Design review of the part built by this model. Coordinates are the model's own, in mm. A direction names the side the tool comes from. Round coordinates to 2 decimals unless told otherwise and drop trailing zeros. Order: outer loops, then holes, each group sorted by start corner. A loop starts at its lowest first (then second) coordinate and runs counter-clockwise, first axis right, second up.
from build123d import *

# Parameters (mm, degrees)
SKETCH1_W = 25
SKETCH1_H = 3
SKETCH4_W = 0.74
SKETCH4_H = 0.5
SKETCH5_W = 0.74
SKETCH5_H = 0.5


with BuildPart() as part:
    # Sketch1 → Revolve1 (revolve)
    with BuildSketch(Plane.XY):
        with Locations((0, 1.5)):
            Rectangle(SKETCH1_W, SKETCH1_H)
    revolve(axis=Axis((12.5, 0, 0), (-1, 0, 0)))

    # Sketch2 → Cut-Revolve1 (revolve, cut)
    with BuildSketch(Plane.XY):
        Polygon((11.75, 3), (12.5, 2.25), (12.5, 3), align=None)
    revolve(axis=Axis((12.5, 0, 0), (-1, 0, 0)), mode=Mode.SUBTRACT)

    # Sketch3 → Cut-Revolve2 (revolve, cut)
    with BuildSketch(Plane.XY):
        Polygon((-12.5, 2.25), (-11.75, 3), (-12.5, 3), align=None)
    revolve(axis=Axis((12.5, 0, 0), (-1, 0, 0)), mode=Mode.SUBTRACT)

    # Sketch4 → Cut-Revolve3 (revolve, cut)
    with BuildSketch(Plane.XY):
        with Locations((9.87, 2.75)):
            Rectangle(SKETCH4_W, SKETCH4_H)
    revolve(axis=Axis((12.5, 0, 0), (-1, 0, 0)), mode=Mode.SUBTRACT)

    # Sketch5 → Cut-Revolve4 (revolve, cut)
    with BuildSketch(Plane.XY):
        with Locations((-9.87, 2.75)):
            Rectangle(SKETCH5_W, SKETCH5_H)
    revolve(axis=Axis((12.5, 0, 0), (-1, 0, 0)), mode=Mode.SUBTRACT)


solid = part.part
1) To check wall thickness, follow line 1 along X through (y, z) = (-2.6, 1.3); line 2 along X through (y, z) = (1.75, -2); line 3 along Z through (x, y) = (-9.25, -2.35). State the ranges of each line that lie inside material, in increasing order.
Results:
line 1: x = -11.84 to -10.24, -9.5 to 9.5, 10.24 to 11.84
line 2: x = -12.09 to -10.24, -9.5 to 9.5, 10.24 to 12.09
line 3: z = -1.86 to 1.86
2) Clearance check with flat-ended pins moving along their axes: P1, Ø1, axis at x = -1, y = 1, coming from the -Z side; P2, Ø1.5, axis at x = -6.5, z = 0.5, coming from the +Y side. State where each tip first meets the part, or that it passes through.
Results:
P1: stops at z = -2.96
P2: stops at y = 3
3) Take a section at C-C on x = 1.25. Give the boundary of the cut face in (y, z).
Results:
outline: circle Ø6 at (0, 0)
4) The part is to be moulded in two halves that separate along X. For faces 3 (the face through (-10.24, 2, -2)), 4 (the face through (12.5, 0, 0)), 5 (the face through (-12.5, 0, 0)), say which applies: released by +X, released by -X, zero draft, split by the parting line, or undercut.
Results:
face 3: undercut
face 4: released by +X
face 5: released by -X
5) Take a section at A-A on z = 0. Give the boundary of the cut face in (x, y).
Results:
outline: (-12.5, -2.25) - (-11.75, -3) - (-10.24, -3) - (-10.24, -2.5) - (-9.5, -2.5) - (-9.5, -3) - (9.5, -3) - (9.5, -2.5) - (10.24, -2.5) - (10.24, -3) - (11.75, -3) - (12.5, -2.25) - (12.5, 2.25) - (11.75, 3) - (10.24, 3) - (10.24, 2.5) - (9.5, 2.5) - (9.5, 3) - (-9.5, 3) - (-9.5, 2.5) - (-10.24, 2.5) - (-10.24, 3) - (-11.75, 3) - (-12.5, 2.25) - close
6) For faces 1 (the face through (0, -3, 0)), 2 (the face through (-9.5, 2, -2)), list the 3-axis set-ups (+Z, -Z, +X, -X, +Y, -Y) from which the entire face can be reached by the end or side of a thin tool; tool diameter is ignored.
Results:
face 1: +X, -X
face 2: none
